from build123d import *

# Parameters (mm, degrees)
ESQUISSE1_R        = 25
BOSS_EXTRU_1_DEPTH = 5
BOSS_EXTRU_2_DEPTH = 10
CONG_2_R           = 5


with BuildPart() as part:
    # Esquisse1 → Boss.-Extru.1 (new body)
    with BuildSketch(Plane.XY):
        Circle(ESQUISSE1_R)
    extrude(amount=BOSS_EXTRU_1_DEPTH)

    # Esquisse2 → Boss.-Extru.2 (add)
    with BuildSketch(Plane.XY.offset(5)):
        with BuildLine():
            Line((-19.732650608, 15.35), (19.732650608, 15.35))
            ThreePointArc((19.732650608, 15.35), (17.308633531, 18.039157555), (14.52162181, 20.35))
            Line((14.52162181, 20.35), (-14.52162181, 20.35))
            ThreePointArc((-14.52162181, 20.35), (-17.308633531, 18.039157555), (-19.732650608, 15.35))
        make_face()
        with BuildLine():
            Line((-14.52162181, -20.35), (14.52162181, -20.35))
            ThreePointArc((14.52162181, -20.35), (17.308633531, -18.039157555), (19.732650608, -15.35))
            Line((19.732650608, -15.35), (-19.732650608, -15.35))
            ThreePointArc((-19.732650608, -15.35), (-17.308633531, -18.039157555), (-14.52162181, -20.35))
        make_face()
    extrude(amount=BOSS_EXTRU_2_DEPTH)

    # Congé2
    # the kernel refuses this fillet: 5 mm, written as the material it adds along each edge
    with BuildSketch(Plane(origin=(27.02162181, 20.35, 5), x_dir=(0, 1, 0), z_dir=(-1, 0, 0))) as cong_2_piece_1_section:
        with BuildLine():
            CenterArc((CONG_2_R, -CONG_2_R), CONG_2_R, 90, 90)
            Line((0, -CONG_2_R), (0, 0))
            Line((0, 0), (CONG_2_R, 0))
        make_face()
    cong_2_piece_1 = extrude(amount=54.043243621, mode=Mode.PRIVATE)
    cong_2_piece_1 = cong_2_piece_1 & Plane(origin=(0, 0, 6.238001242), x_dir=(1, 0, 0), z_dir=(0, 0, -1)) * Cylinder(25, 129, mode=Mode.PRIVATE)
    add(cong_2_piece_1)
    with BuildSketch(Plane(origin=(-27.02162181, -20.35, 5), x_dir=(0, -1, 0), z_dir=(1, 0, 0))) as cong_2_piece_2_section:
        with BuildLine():
            CenterArc((CONG_2_R, -CONG_2_R), CONG_2_R, 90, 90)
            Line((0, -CONG_2_R), (0, 0))
            Line((0, 0), (CONG_2_R, 0))
        make_face()
    cong_2_piece_2 = extrude(amount=54.043243621, mode=Mode.PRIVATE)
    cong_2_piece_2 = cong_2_piece_2 & Plane(origin=(0, 0, 6.238012691), x_dir=(1, 0, 0), z_dir=(0, 0, -1)) * Cylinder(25, 129, mode=Mode.PRIVATE)
    add(cong_2_piece_2)


solid = part.part
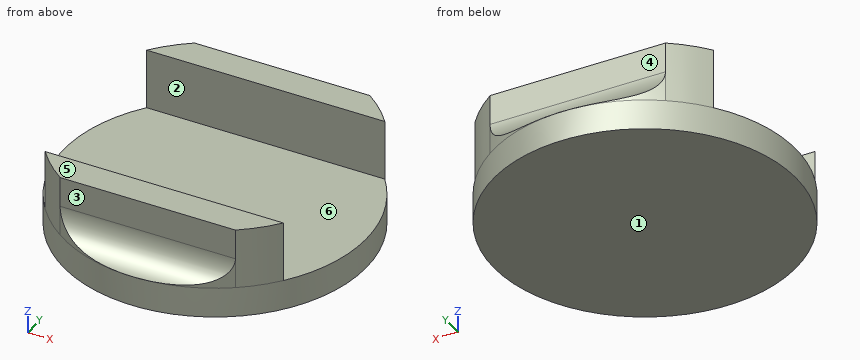
Input: part model. Units: mm. Frame: model coordinates. Face numbers are marked on the shaded views. A direction names the side the tool comes from. Coordinates: 2 decimals unless noted, no trailing zeros. Order: outer loops, then holes, each group sorted by start corner. A loop starts at its lowest first (then second) coordinate and runs counter-clockwise, first axis right, second up. Notation, with made-up numbers: M 79,25.5 L 109,25.5 A20 cw 109,32.5 Z; hole C -23.75,-37 d6. An arc over 180 degrees is marked long. Answer in a Markdown table with one row per item.
(1) Material intervals for line 1 (Y direction, x = 9, z = 13); line 2 (Z direction, x = 1.5, y = 13.5), sorted ascending. Write a range as [from, to].
Numbers:
| item | result |
|---|---|
| line 1 | y = [-20.35, -15.35], [15.35, 20.35] |
| line 2 | z = [0, 5] |
(2) Section query D-D, the plane z = 6. Output: boundary loops of the cut face in (x, y), plus the area to 3 significant figures.
Numbers:
| item | result |
|---|---|
| outline | M -19.73,-15.35 A25 ccw -11.2,-22.35 L 11.2,-22.35 A25 ccw 19.73,-15.35 Z; M -19.73,15.35 L 19.73,15.35 A25 ccw 11.2,22.35 L -11.2,22.35 A25 ccw Z |
| area | 451 mm^2 |
(3) Section query C-C, the plane y = 0. Output: boundary loops of the cut face in (x, z), plus the area to 3 significant figures.
Numbers:
| item | result |
|---|---|
| outline | M -25,0 L 25,0 L 25,5 L -25,5 Z |
| area | 250 mm^2 |
(4) Section query A-A, the plane z = 13.5. Output: boundary loops of the cut face in (x, y), plus the area to 3 significant figures.
Numbers:
| item | result |
|---|---|
| outline | M -19.73,-15.35 A25 ccw -14.52,-20.35 L 14.52,-20.35 A25 ccw 19.73,-15.35 Z; M -19.73,15.35 L 19.73,15.35 A25 ccw 14.52,20.35 L -14.52,20.35 A25 ccw Z |
| area | 348 mm^2 |
(5) Contact query for flat-ended pins moving along their axis: pin 1 Ø1.5 at (x, y) = (19.5, -14) entering from -Z; pin 2 Ø5 at (x, z) = (10, 9) entering from +Y; pin 3 Ø3 at (y, z) = (-12, 4.5) entering from -X; pin 4 Ø1 at (x, z) = (-14, 10.5) entering from -Y. Output: stop coordinate, or through.
Numbers:
| item | result |
|---|---|
| pin 1 | stops at z = 0 |
| pin 2 | stops at y = 21.78 |
| pin 3 | stops at x = -22.69 |
| pin 4 | stops at y = -20.35 |
(6) Section query B-B, the plane x = 0. Output: boundary loops of the cut face in (y, z), plus the area to 3 significant figures.
Numbers:
| item | result |
|---|---|
| outline | M -25,0 L 25,0 L 25,5.01 A5 cw 20.35,10 L 20.35,15 L 15.35,15 L 15.35,5 L -15.35,5 L -15.35,15 L -20.35,15 L -20.35,10 A5 cw -25,5.01 Z |
| area | 361 mm^2 |
(7) Access query for the marked faces 1, 2 and 3. Directions: +Z, -Z, +X, -X, +Y, -Y. A direction counts if a zero-diameter tool reaches every point of the face in a straight line with its end or side. Return the directions, or none.
Numbers:
| item | result |
|---|---|
| face 1 | -Z, +X, -X, +Y, -Y |
| face 2 | +Z, +X, -X |
| face 3 | +Z, +X, -X, -Y |
(8) Draft query along Y for the marked faces 4, 5 and 6. Return one class per face: pulls with the +Y half, pulls with the -Y half, needs draft (parallel to the pull), parting line crosses it, or undercut.
Numbers:
| item | result |
|---|---|
| face 4 | pulls with the +Y half |
| face 5 | needs draft |
| face 6 | undercut |
